Part model, mm, in its own coordinate system. Face numbers are marked on the shaded views. A direction names the side the tool comes from. Give positions to 0.01 mm unless a question says otherwise; leave off trailing zeros. Loops run counter-clockwise (first coordinate to the right, second up) from the corner with the lowest first, then second, coordinate; pieces in that order, holes last. Notation, with made-up numbers: (-11, -4) -> (33, -4) arc R32 cw to (33, 28) -> close; hole circle Ø5 at (6, 49). An arc over 180 degrees is marked (long way). One line per question, with ' | ' between items.
```python
from build123d import *

# Parameters (mm, degrees)
BOSS_EXTRUDE1_DEPTH = 120
CUT_EXTRUDE2_DEPTH  = 2
CUT_EXTRUDE3_START  = -2
CUT_EXTRUDE3_DEPTH  = 2


with BuildPart() as part:
    # Sketch1 → Boss-Extrude1 (new body)
    with BuildSketch(Plane(origin=(0, 0, 0), x_dir=(1, 0, 0), z_dir=(0, 1, 0))):
        Polygon((0, 0), (0, 1050), (300, 1050), (600, 650), (600, 0), (598, 0), (598, 649.333333333), (299, 1048), (2, 1048), (2, 0), align=None)
    extrude(amount=BOSS_EXTRUDE1_DEPTH)

    # Sketch7 → Cut-Extrude2 (cut)
    with BuildSketch(Plane(origin=(600, 0, 0), x_dir=(0, 0, -1), z_dir=(1, 0, 0))):
        with BuildLine():
            Line((45, 20), (45, 35))
            ThreePointArc((45, 35), (50, 40), (55, 35))
            Line((55, 35), (55, 20))
            ThreePointArc((55, 20), (50, 15), (45, 20))
        make_face()
        with BuildLine():
            Line((75, 20), (75, 35))
            ThreePointArc((75, 35), (80, 40), (85, 35))
            Line((85, 35), (85, 20))
            ThreePointArc((85, 20), (80, 15), (75, 20))
        make_face()
        with BuildLine():
            Line((195, 20), (195, 35))
            ThreePointArc((195, 35), (200, 40), (205, 35))
            Line((205, 35), (205, 20))
            ThreePointArc((205, 20), (200, 15), (195, 20))
        make_face()
        with BuildLine():
            Line((225, 20), (225, 35))
            ThreePointArc((225, 35), (230, 40), (235, 35))
            Line((235, 35), (235, 20))
            ThreePointArc((235, 20), (230, 15), (225, 20))
        make_face()
    extrude(amount=-CUT_EXTRUDE2_DEPTH, mode=Mode.SUBTRACT)

    # Sketch8 → Cut-Extrude3 (cut)
    with BuildSketch(Plane.ZY.offset(CUT_EXTRUDE3_START)):
        with BuildLine():
            Line((-45, 35), (-45, 20))
            ThreePointArc((-45, 20), (-50, 15), (-55, 20))
            Line((-55, 20), (-55, 35))
            ThreePointArc((-55, 35), (-50, 40), (-45, 35))
        make_face()
        with BuildLine():
            Line((-75, 35), (-75, 20))
            ThreePointArc((-75, 20), (-80, 15), (-85, 20))
            Line((-85, 20), (-85, 35))
            ThreePointArc((-85, 35), (-80, 40), (-75, 35))
        make_face()
        with BuildLine():
            Line((-395, 35), (-395, 20))
            ThreePointArc((-395, 20), (-400, 15), (-405, 20))
            Line((-405, 20), (-405, 35))
            ThreePointArc((-405, 35), (-400, 40), (-395, 35))
        make_face()
        with BuildLine():
            Line((-425, 35), (-425, 20))
            ThreePointArc((-425, 20), (-430, 15), (-435, 20))
            Line((-435, 20), (-435, 35))
            ThreePointArc((-435, 35), (-430, 40), (-425, 35))
        make_face()
        with BuildLine():
            Line((-745, 35), (-745, 20))
            ThreePointArc((-745, 20), (-750, 15), (-755, 20))
            Line((-755, 20), (-755, 35))
            ThreePointArc((-755, 35), (-750, 40), (-745, 35))
        make_face()
        with BuildLine():
            Line((-775, 35), (-775, 20))
            ThreePointArc((-775, 20), (-780, 15), (-785, 20))
            Line((-785, 20), (-785, 35))
            ThreePointArc((-785, 35), (-780, 40), (-775, 35))
        make_face()
    extrude(amount=CUT_EXTRUDE3_DEPTH, mode=Mode.SUBTRACT)


solid = part.part
```
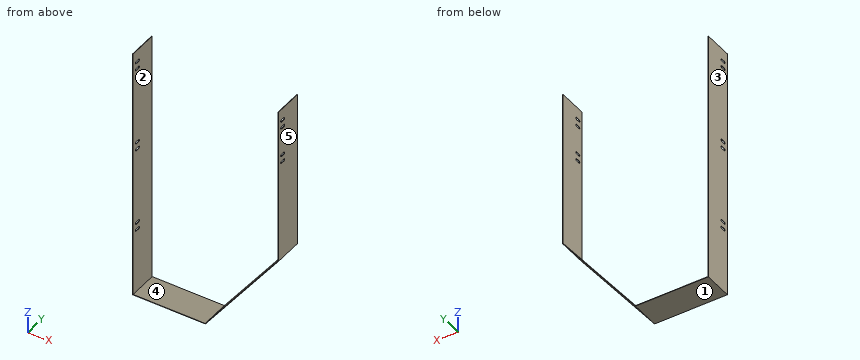
1) Tool access for the marked faces 4 and 5: list every direction of +Z, -Z, +X, -X, +Y, -Y with a clear straight run to the whole face (end or side of a thin tool).
Found:
face 4: +Z, +Y, -Y | face 5: +Z, -Z, +X, +Y, -Y
2) Saw through at A-A (z = -337.5). Give the cut face in (x, y).
Found:
outline: (0, 0) -> (2, 0) -> (2, 120) -> (0, 120) -> close; (598, 0) -> (600, 0) -> (600, 120) -> (598, 120) -> close
3) Pull direction X, two halves, no side cores. Call the marked faces 1, 2 and 3: pulls with the +X half, pulls with the -X half, needs draft (parallel to the pull), parting line crosses it, or undercut.
Found:
face 1: needs draft | face 2: undercut | face 3: pulls with the -X half
4) Saw through at B-B (y = 63). Give the cut face in (x, z), and give its area (3 significant figures).
Found:
outline: (0, -1050) -> (300, -1050) -> (600, -650) -> (600, 0) -> (598, 0) -> (598, -649.33) -> (299, -1048) -> (2, -1048) -> (2, 0) -> (0, 0) -> close | area: 4,990 mm2
5) Saw through at D-D (x = 232). Give the cut face in (y, z).
Found:
outline: (0, -1050) -> (120, -1050) -> (120, -1048) -> (0, -1048) -> close
6) Drill centre lines: line 1 (X direction, y = 81.5, z = -353.5); line 2 (Z direction, x = 164.5, y = 26.5); line 3 (X direction, y = 59, z = -677). Where is each one in solid material? Low to high.
Found:
line 1: 0 to 2, 598 to 600 | line 2: -1050 to -1048 | line 3: 0 to 2, 577.25 to 579.75
7) Saw through at C-C (z = -951.5). Give the cut face in (x, y) (3 decimals).
Found:
outline: (0, 0) -> (2, 0) -> (2, 120) -> (0, 120) -> close; (371.375, 0) -> (373.875, 0) -> (373.875, 120) -> (371.375, 120) -> close
8) Pin check, flat tips, straight feed: P1, Ø0.6, axis at x = 599, y = 28, coming from the -Z side; P2, Ø2, axis at x = 599, y = 27, coming from the -Z side; P3, Ø1.5, axis at x = 349.5, y = 31, coming from the -Z side. Stop position of each tip, or through.
Found:
P1: z = -651.73 | P2: z = -652.67 | P3: z = -985
